Design review of the part built by this model. Coordinates are the model's own, in mm. A direction names the side the tool comes from. Give positions to 0.01 mm unless a question says otherwise; leave off trailing zeros. Write each loop counter-clockwise with the first axis right and the second up, starting at its lowest first coordinate (ties: lowest second). Pieces come first, ordered by that corner, then holes. Notation, with made-up numbers: (31.25, -10) -> (40.25, -10) arc R10 ccw to (40.25, 7) -> close; hole circle Ø7 at (77, 28). An arc over 180 degrees is marked (long way). Use CSV: the item, a comma, the result in double quotes.
```python
from build123d import *

# Parameters (mm, degrees)
F0_W     = 60
F0_H     = 15
F1_DEPTH = 5
F3_DEPTH = 15
F4_DEPTH = 5
F6_D     = 5.5


with BuildPart() as f1:
    # F0 (on Top) → F1 (new body)
    with BuildSketch(Plane.XY):
        Rectangle(F0_W, F0_H)
        with BuildLine():
            Line((-30, -7.5), (-30, 7.5))
            ThreePointArc((-30, 7.5), (-37.5, 0), (-30, -7.5))
        make_face()
        with BuildLine():
            ThreePointArc((30, -7.5), (37.5, 0), (30, 7.5))
            Line((30, 7.5), (30, -7.5))
        make_face()
    extrude(amount=F1_DEPTH)

    # F2 (on face) → F3 (join)
    with BuildSketch(Plane.XZ.offset(7.5)):
        with BuildLine():
            Line((20.5, 23.5), (18.5, 23.5))
            ThreePointArc((18.5, 23.5), (13.0814754325, 10.4185245286), (-5.51e-08, 5))
            Line((-5.51e-08, 5), (8.8317608663, 5))
            ThreePointArc((8.8317608663, 5), (17.3392776343, 12.5638466031), (20.5, 23.5))
        make_face()
        with BuildLine():
            ThreePointArc((-5.51e-08, 5), (-13.0814754714, 10.4185245675), (-18.5, 23.5))
            Line((-18.5, 23.5), (-20.5, 23.5))
            ThreePointArc((-20.5, 23.5), (-17.3392776343, 12.5638466031), (-8.8317608663, 5))
            Line((-8.8317608663, 5), (-5.51e-08, 5))
        make_face()
        with BuildLine():
            Line((20.5, 5), (20.5, 23.5))
            ThreePointArc((20.5, 23.5), (17.3392776343, 12.5638466031), (8.8317608663, 5))
            Line((8.8317608663, 5), (20.5, 5))
        make_face()
        with BuildLine():
            ThreePointArc((-8.8317608663, 5), (-17.3392776343, 12.5638466031), (-20.5, 23.5))
            Line((-20.5, 23.5), (-20.5, 5))
            Line((-20.5, 5), (-8.8317608663, 5))
        make_face()
    extrude(amount=-F3_DEPTH)

    # F2 (on face) → F4 (join)
    with BuildSketch(Plane.XZ.offset(7.5)):
        with BuildLine():
            ThreePointArc((-5.51e-08, 5), (13.0814754325, 10.4185245286), (18.5, 23.5))
            Line((18.5, 23.5), (15, 23.5))
            ThreePointArc((15, 23.5), (0, 8.5), (-15, 23.5))
            Line((-15, 23.5), (-18.5, 23.5))
            ThreePointArc((-18.5, 23.5), (-13.0814754714, 10.4185245675), (-5.51e-08, 5))
        make_face()
    extrude(amount=-F4_DEPTH)

    # F6 (through all)
    with Locations(Plane.XY.offset(5)):
        with Locations((30, 0), (-30, 0)):
            Hole(F6_D / 2)


solid = f1.part
```
(1) Mouldability with a two-part tool opening along Y and no side actions: class faces 1 (the face through (0, 7.5, 4)), 2 (the face through (-37.5, 0.16, 2.46)), 3 (the face through (0, -7.5, 7)), 4 (the face through (32.747, 0.121, 2.465)) as +Y half, -Y half, draft (parallel to the pull), parting line (faces both ways), or undercut.
Established:
face 1,"+Y half"
face 2,"parting line"
face 3,"-Y half"
face 4,"undercut"
(2) Tool access review of faces 5 (the face through (-20.5, 0, 14)), 6 (the face through (0, 2, 5)), 7 (the face through (-27.253, 0.121, 2.465)), 8 (the face through (27, 0, 5)), 9 (the face through (-19, -2, 23.5)): name each direction out of +Z, -Z, +X, -X, +Y, -Y from which nothing blocks a thin tool from reaching the whole face with its end or side.
Established:
face 5,"+Z, -X, +Y, -Y"
face 6,"+Z, +Y"
face 7,"+Z, -Z"
face 8,"+Z, +X, +Y, -Y"
face 9,"+Z, +X, -X, +Y, -Y"
(3) Take a section at A-A (y = 0). Write out the cut boundary in (x, z).
Established:
outline,"(-37.5, 0) -> (-32.75, 0) -> (-32.75, 5) -> (-37.5, 5) -> close; (-27.25, 0) -> (27.25, 0) -> (27.25, 5) -> (20.5, 5) -> (20.5, 23.5) -> (18.5, 23.5) arc R18.5 cw to (-18.5, 23.5) -> (-20.5, 23.5) -> (-20.5, 5) -> (-27.25, 5) -> close; (32.75, 0) -> (37.5, 0) -> (37.5, 5) -> (32.75, 5) -> close"
(4) For line 1 along Y through (x, z) = (30, 1.45); line 2 along Z through (x, y) = (-0.5, -4.75); line 3 along Y through (x, z) = (-11.5, 13), list the stretches that pass through material, from the lowest coordinate up. Write a range as [from, to].
Established:
line 1,"y = [-7.5, -2.75], [2.75, 7.5]"
line 2,"z = [0, 8.51]"
line 3,"y = [-7.5, -2.5]"
(5) Clearance check with flat-ended pins moving along their axes: pin 1 (9.5 mm diameter, centred on x = 1, z = 16.5, fed in from +Y); pin 2 (6 mm diameter, centred on y = -2.5, z = 13.5, fed in from -X); pin 3 (7.5 mm diameter, centred on y = 3, z = 14.5, fed in from +X); pin 4 (1.5 mm diameter, centred on x = -22, y = 2, fed in from +Z). State where each tip first meets the part, or that it passes through.
Established:
pin 1,"passes through"
pin 2,"stops at x = -20.5"
pin 3,"stops at x = 20.5"
pin 4,"stops at z = 5"
(6) Take a section at D-D (y = 4.25). Write out the cut boundary in (x, z).
Established:
outline,"(-36.18, 0) -> (36.18, 0) -> (36.18, 5) -> (20.5, 5) -> (20.5, 23.5) -> (18.5, 23.5) arc R18.5 cw to (-18.5, 23.5) -> (-20.5, 23.5) -> (-20.5, 5) -> (-36.18, 5) -> close"
(7) Take a section at B-B (z = 19.5). Write out the cut boundary in (x, y).
Established:
outline,"(-20.5, -7.5) -> (-14.46, -7.5) -> (-14.46, -2.5) -> (-18.06, -2.5) -> (-18.06, 7.5) -> (-20.5, 7.5) -> close; (14.46, -7.5) -> (20.5, -7.5) -> (20.5, 7.5) -> (18.06, 7.5) -> (18.06, -2.5) -> (14.46, -2.5) -> close"
(8) Take a section at C-C (z = 2.75). Write out the cut boundary in (x, y).
Established:
outline,"(-30, -7.5) -> (30, -7.5) arc R7.5 ccw to (30, 7.5) -> (-30, 7.5) arc R7.5 ccw to start; hole circle Ø5.5 at (-30, 0); hole circle Ø5.5 at (30, 0)"
